Study the drawing (mm; zero at the part's minimum x, y, z) and answer. Give positions to 0.01 mm unless a question says otherwise; leave off trailing zeros. Loops run counter-clockwise (first coordinate to the right, second up) from the corner with the lowest first, then second, coordinate; pieces in that order, holes last. Notation, with made-up numbers: M 42.25,17.25 L 95.25,17.25 A26 cw 95.25,32.25 Z; hole C -0.75,35.5 d1. An arc over 180 degrees is marked long. Use one line per item in the form item = value. Start each with the question number.
1. Each of these flat-tipped pins is pushed along its axis until it touches: pin 1 Ø1.8 at (x, y) = (2.5, 38.5) entering from -Z; pin 2 Ø6 at (x, z) = (70, 21) entering from +Y; pin 3 Ø1 at (x, z) = (30.5, 71) entering from +Y; pin 4 Ø1 at (x, y) = (38, 21.5) entering from -Z. Where does it stop, or does it pass through?
2. The part is cut by section B-B (z = 14.5). Write down the section's boundary in (x, y), and give its area (3 significant figures).
3. The part is cut by section A-A (x = 47.5). Write down the section's boundary in (y, z).
4. Straight lines are drawn through the part: line 1 (Z direction, x = 65, y = 4); line 2 (X direction, y = 1.3, z = 36); line 3 (Y direction, x = 2.5, z = 26.5). For each, find the intervals that lie inside material, in ascending order. Write a range as from..to.
5. The mould has two halves that part along Z. Classify the marked faces 1, 2, 3 and 4: released by +Z, released by -Z, zero draft, split by the parting line, or undercut.
6. The part is cut by section C-C (y = 22). Write down the section's boundary in (x, z), and give its area (3 significant figures).
7. The part is cut by section D-D (x = 14). Write down the section's boundary in (y, z), and give its area (3 significant figures).
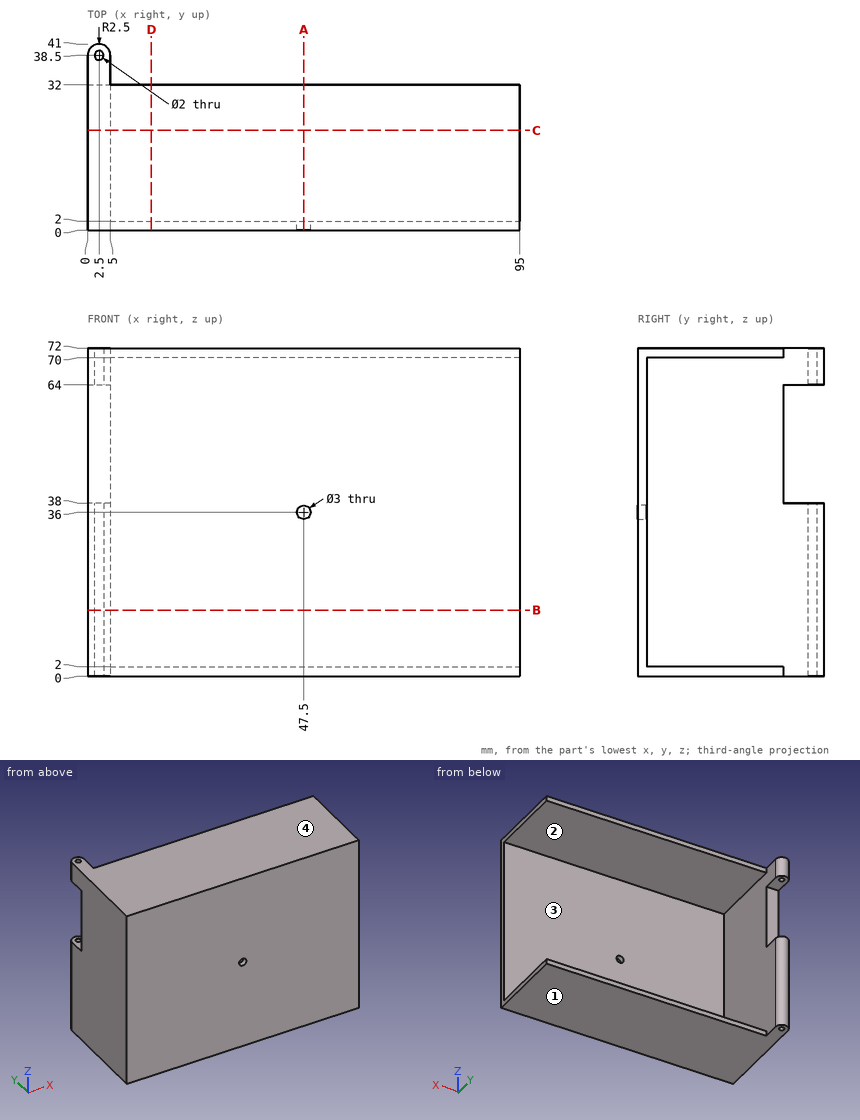
Derived:
q1.pin_1 = through
q1.pin_2 = 2
q1.pin_3 = 32
q1.pin_4 = 0
q2.outline = M 0,0 L 95,0 L 95,2 L 5,2 L 5,38.5 A2.5 ccw 0,38.5 Z; hole C 2.5,38.5 d2
q2.area = 379 mm2
q3.outline = M 0,0 L 32,0 L 32,2 L 2,2 L 2,34.5 L 0,34.5 Z; M 0,37.5 L 2,37.5 L 2,70 L 32,70 L 32,72 L 0,72 Z
q4.line_1 = 0..2, 70..72
q4.line_2 = 0..46, 49..95
q4.line_3 = 0..37.5, 39.5..41
q5.face_1 = released by -Z
q5.face_2 = undercut
q5.face_3 = undercut
q5.face_4 = released by +Z
q6.outline = M 0,0 L 95,0 L 95,2 L 5,2 L 5,70 L 95,70 L 95,72 L 0,72 Z
q6.area = 720 mm2
q7.outline = M 0,0 L 32,0 L 32,2 L 2,2 L 2,70 L 32,70 L 32,72 L 0,72 Z
q7.area = 264 mm2
